```python
from build123d import *

# Parameters (mm, degrees)
F0_R     = 19.05
F1_DEPTH = 203.2
F3_DEPTH = 25.4
F4_DEPTH = 25.4
F5_R     = 15.5892770942


with BuildPart() as f1:
    # F0 (on Top) → F1 (new body)
    with BuildSketch(Plane.XY):
        Circle(F0_R)
    extrude(amount=F1_DEPTH)

    # F2 (on face) → F3 (cut)
    with BuildSketch(Plane.XY.offset(203.2)):
        with BuildLine():
            Line((-12.2428, -14.5950795873), (-12.2428, 14.5950795873))
            ThreePointArc((-12.2428, 14.5950795873), (-19.05, 0), (-12.2428, -14.5950795873))
        make_face()
    extrude(amount=-F3_DEPTH, mode=Mode.SUBTRACT)

    # F2 (on face) → F4 (cut)
    with BuildSketch(Plane.XY.offset(203.2)):
        with BuildLine():
            ThreePointArc((13.6144, -13.3248119176), (17.6388324444, -7.1954214609), (19.05, 0))
            ThreePointArc((19.05, 0), (17.6388324444, 7.1954214609), (13.6144, 13.3248119176))
            Line((13.6144, 13.3248119176), (13.6144, -13.3248119176))
        make_face()
    extrude(amount=-F4_DEPTH, mode=Mode.SUBTRACT)

    # F5
    f5_edges = [f1.edges().sort_by_distance(p)[0] for p in [
        (-19.05, 0, 0),
    ]]
    fillet(f5_edges, radius=F5_R)


solid = f1.part
```
Build history of the part. All positions in model axes, mm. A direction names the side the tool comes from. Give positions to 0.01 mm unless a question says otherwise; leave off trailing zeros. Loops run counter-clockwise (first coordinate to the right, second up) from the corner with the lowest first, then second, coordinate; pieces in that order, holes last. Notation, with made-up numbers: (73, 49) -> (113, 49) arc R27 ccw to (113, 76) -> close; hole circle Ø10 at (-2.75, -30). An arc over 180 degrees is marked (long way). One line per question, with ' | ' between items. Start each with the question number.
1) 3-axis set-ups, long thin cutter, end or side, ignore diameter. For faces 1 (the flat face through (16, 0, 177.8)), 2 (the flat face through (1, 0, 203.2)), 3 (the flat face through (-12.243, 0, 191)): which of +Z, -Z, +X, -X, +Y, -Y reach the whole face in a straight line?
2) Cut at A-A (z = 32). Give the cut face in (x, y).
3) Probe L1, parallel to Y at x = 0.5, z = 63; L2, parallel to X at y = 1, z = 111; L3, parallel to Z at x = 8.5, y = 7. List the from-to ranges inside material, lowest first.
4) Pin check, flat tips, straight feed: pin 1 (2 mm diameter, centred on x = 10.5, y = -12.5, fed in from -Z); pin 2 (1.5 mm diameter, centred on x = 3, z = 94.5, fed in from -Y); pin 3 (5 mm diameter, centred on x = 4, z = 94.5, fed in from +Y). Stop position of each tip, or through.
Return value:
1) face 1: +Z, +X, +Y, -Y | face 2: +Z, +X, -X, +Y, -Y | face 3: +Z, -X, +Y, -Y
2) outline: circle Ø38.1 at (0, 0)
3) L1: -19.04 to 19.04 | L2: -19.02 to 19.02 | L3: 1.95 to 203.2
4) pin 1: z = 5.48 | pin 2: y = -18.92 | pin 3: y = 18.99
